Work out the finished part from the listing and answer in its coordinate system (mm). Coordinates: 2 decimals unless noted, no trailing zeros. Write each loop counter-clockwise with the first axis right and the second up, starting at its lowest first coordinate (ties: lowest second). Pieces come first, ordered by that corner, then holes. Notation, with made-up numbers: M 78,59.25 L 84,59.25 A26 cw 84,82.25 Z; hole C 25,-38.5 d8. An arc over 180 degrees is marked long. Answer as CSV lines item,"result". Start each with the question number.
(1) A cutting plane is placed at A-A on y = 12. Give the vertices of the cut face in (x, z).
(2) A cutting plane is placed at D-D on y = 58. Give the vertices of the cut face in (x, z).
(3) Find the intervals of material crossed by L1, parallel to X at y = 45.5, z = 0.55; L2, parallel to X at y = 39, z = 1.4; L3, parallel to Y at x = 62.5, z = 2.35, in increasing order. Write a range as [from, to].
(4) A cutting plane is placed at C-C on z = 0.6. Count the separate pieces of the cut face and the enclosed holes in it, then the cut area to 3 significant figures.
(5) A cutting plane is placed at B-B on x = 55.5. Give the vertices of the cut face in (y, z).
(6) Flat-ended cylindrical pins translate along their axes: P1, Ø0.9, axis at y = 14.5, z = 1.5, coming from the -X side; P2, Ø1.5, axis at y = 65, z = 1, coming from the +X side; P3, Ø1.5, axis at x = 125, z = 1.5, coming from the -Y side. Find the tip coordinate at first contact, or state that the pin passes through.
Autodesk Inventor part; units mm, degrees
ref_plane "YZ Plane" through (0, 0, 0) normal (1, 0, 0) x (0, 1, 0)
ref_plane "XZ Plane" through (0, 0, 0) normal (0, 1, 0) x (-1, 0, 0)
ref_plane "XY Plane" through (0, 0, 0) normal (0, 0, 1) x (1, 0, 0)
sketch "Sketch1" plane through (0, 0, 0) normal (0, 0, 1) x (1, 0, 0)
  line L0 (0, 0) -> (3, 0)
  line L1 (3, 0) -> (123, 0)
  line L2 (0, 0) -> (0, 3)
  line L3 (0, 3) -> (3, 3)
  line L4 (3, 3) -> (3, 23)
  line L5 (3, 23) -> (0, 23)
  line L6 (0, 23) -> (0, 43)
  line L7 (0, 43) -> (3, 43)
  line L8 (3, 43) -> (3, 63)
  line L9 (3, 63) -> (3, 66)
  line L10 (3, 66) -> (23, 66)
  line L11 (23, 66) -> (23, 63)
  line L12 (23, 63) -> (43, 63)
  line L13 (43, 63) -> (43, 66)
  line L14 (43, 66) -> (63, 66)
  line L15 (63, 66) -> (63, 63)
  line L16 (63, 63) -> (83, 63)
  line L17 (83, 63) -> (83, 66)
  line L18 (83, 66) -> (103, 66)
  line L19 (103, 66) -> (103, 63)
  line L20 (103, 63) -> (123, 63)
  line L21 (123, 63) -> (126, 63)
  line L22 (126, 63) -> (126, 43)
  line L23 (126, 43) -> (123, 43)
  line L24 (123, 43) -> (123, 23)
  line L25 (123, 23) -> (126, 23)
  line L26 (126, 23) -> (126, 3)
  line L27 (126, 3) -> (123, 3)
  line L28 (123, 0) -> (123, 3)
  dimension "d0" = 3
  dimension "d1" = 120
  dimension "d2" = 3
  dimension "d3" = 20
  dimension "d4" = 20
  dimension "d5" = 20
  dimension "d6" = 3
  dimension "d7" = 20
  dimension "d8" = 20
  dimension "d9" = 20
  dimension "d10" = 20
  dimension "d11" = 20
  dimension "d12" = 20
  dimension "d13" = 3
  dimension "d14" = 20
  dimension "d15" = 20
  dimension "d16" = 20
extrude "Extrusion1" add sketch "Sketch1" along normal blind 3
sketch "Sketch2" plane through (0, 0, 3) normal (0, 0, 1) x (1, 0, 0)
  line L0 (40, 20) -> (80, 20)
  line L1 (80, 20) -> (80, 5)
  line L2 (80, 5) -> (40, 5)
  line L3 (40, 5) -> (40, 20)
  line L4 (0, 0) -> (123, 0)
  line L5 (8, 51) -> (20, 51)
  line L6 (20, 51) -> (20, 31)
  line L7 (20, 31) -> (8, 31)
  line L8 (8, 31) -> (8, 51)
  line L9 (43, 63) -> (23, 63)
  line L10 (3, 23) -> (3, 3)
  dimension "d19" = 40
  dimension "d20" = 15
  dimension "d21" = 5
  dimension "d22" = 40
  dimension "d26" = 12
  dimension "d27" = 20
  dimension "d28" = 12
  dimension "d29" = 5
extrude "Extrusion2" cut sketch "Sketch2" against normal up to next
fillet "Fillet1" radius 4 8 edges at (20, 31, 1.5) (20, 51, 1.5) (8, 51, 1.5) (8, 31, 1.5) (80, 5, 1.5) (80, 20, 1.5) (40, 20, 1.5) (40, 5, 1.5)
properties part number "ControlBoxFanFace" material "Wood (Birch)"
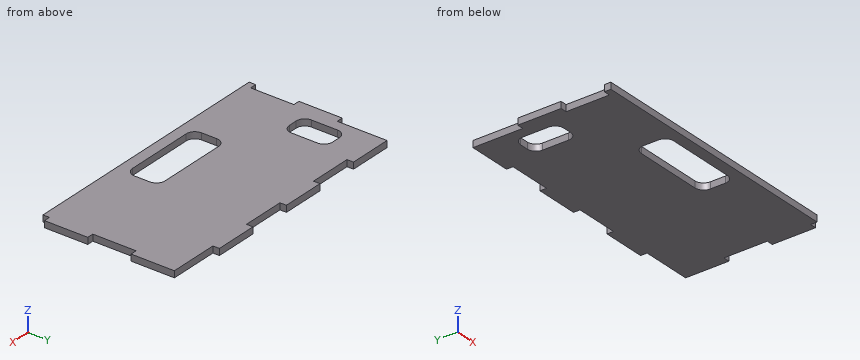
Here are the results:
1,outline,"M 3,0 L 40,0 L 40,3 L 3,3 Z; M 80,0 L 126,0 L 126,3 L 80,3 Z"
2,outline,"M 3,0 L 126,0 L 126,3 L 3,3 Z"
3,L1,"x = [3, 8], [20, 126]"
3,L2,"x = [0, 8], [20, 123]"
3,L3,"y = [0, 5], [20, 66]"
4,separate pieces,"1"
4,enclosed holes,"2"
4,area,"7,120 mm^2"
5,outline,"M 0,0 L 5,0 L 5,3 L 0,3 Z; M 20,0 L 66,0 L 66,3 L 20,3 Z"
6,P1,"stops at x = 3"
6,P2,"stops at x = 103"
6,P3,"stops at y = 3"
